Here's how the part is built. I have some questions about the finished solid (model axes, mm). A direction names the side the tool comes from. Round coordinates to 2 decimals unless told otherwise and drop trailing zeros. Order: outer loops, then holes, each group sorted by start corner. A loop starts at its lowest first (then second) coordinate and runs counter-clockwise, first axis right, second up. Notation, with made-up numbers: (31, 60) -> (75, 60) arc R26 cw to (75, 95) -> close; hole circle Ø4 at (24.25, 15.25). An arc over 180 degrees is marked (long way). Use a Markdown table: item, result. Add a question column.
from build123d import *

# Parameters (mm, degrees)
ESQUISSE11_R                 = 10
ENL_V_MAT_EXTRU_4_DEPTH      = 6.2
ESQUISSE12_R                 = 1.65
ENL_V_MAT_EXTRU_5_DEPTH      = 66.664775353
ESQUISSE14_R                 = 2.85
ENL_V_MAT_EXTRU_8_DEPTH      = 3.6
R_P_TITION_CIRCULAIRE7_COUNT = 3


with BuildPart() as part:
    # Esquisse1 → Révolution1 (revolve)
    with BuildSketch(Plane.XY, mode=Mode.PRIVATE) as r_volution1_sk:
        with BuildLine():
            Line((-45.5, 158.120727786), (-45.5, 145.030169275))
            ThreePointArc((-45.5, 145.030169275), (-23.015367368, 150.247438797), (0, 152))
            Line((0, 152), (0, 158.120727786))
            Line((0, 158.120727786), (-45.5, 158.120727786))
        make_face()
    revolve(r_volution1_sk.sketch.rotate(Axis((0, 0, 0), (0, 1, 0)), 270), axis=Axis((0, 0, 0), (0, 1, 0)))

    # Esquisse11 → Enlèv. mat.-Extru.4 (cut)
    with BuildSketch(Plane(origin=(0, 158.120727786, 0), x_dir=(1, 0, 0), z_dir=(0, 1, 0))):
        with Locations(Location((0, 35, 0), (0, 0, 270))):
            Circle(ESQUISSE11_R)
    enl_v_mat_extru_4 = extrude(amount=-ENL_V_MAT_EXTRU_4_DEPTH, mode=Mode.SUBTRACT)

    # Esquisse12 → Enlèv. mat.-Extru.5 (cut, through all)
    with BuildSketch(Plane(origin=(0, 158.120727786, 0), x_dir=(1, 0, 0), z_dir=(0, 1, 0))):
        with Locations(Location((-30.310889132, 17.5, 0), (0, 0, 270))):
            Circle(ESQUISSE12_R)
    enl_v_mat_extru_5 = extrude(amount=-ENL_V_MAT_EXTRU_5_DEPTH, mode=Mode.SUBTRACT)

    # Esquisse14 → Enlèv. mat.-Extru.8 (cut)
    with BuildSketch(Plane(origin=(0, 147.120727786, 0), x_dir=(1, 0, 0), z_dir=(0, 1, 0))):
        with Locations(Location((-30.310889132, 17.5, 0), (0, 0, 134.033255464))):
            Circle(ESQUISSE14_R)
    enl_v_mat_extru_8 = extrude(amount=ENL_V_MAT_EXTRU_8_DEPTH, mode=Mode.SUBTRACT)

    # Répétition circulaire7: Enlèv. mat.-Extru.4, Enlèv. mat.-Extru.5, Enlèv. mat.-Extru.8 ×3 about axis
    r_p_tition_circulaire7_axis = Axis((0, 0, 0), (0, 1, 0))
    add([enl_v_mat_extru_4.rotate(r_p_tition_circulaire7_axis, i * 360 / R_P_TITION_CIRCULAIRE7_COUNT) for i in range(1, R_P_TITION_CIRCULAIRE7_COUNT)], mode=Mode.SUBTRACT)
    add([enl_v_mat_extru_5.rotate(r_p_tition_circulaire7_axis, i * 360 / R_P_TITION_CIRCULAIRE7_COUNT) for i in range(1, R_P_TITION_CIRCULAIRE7_COUNT)], mode=Mode.SUBTRACT)
    add([enl_v_mat_extru_8.rotate(r_p_tition_circulaire7_axis, i * 360 / R_P_TITION_CIRCULAIRE7_COUNT) for i in range(1, R_P_TITION_CIRCULAIRE7_COUNT)], mode=Mode.SUBTRACT)


solid = part.part
(1) I'm going to push flat-ended pins straight in: P1, Ø1, axis at x = -18, y = 153, coming from the +Z side; P2, Ø1.5, axis at x = 6.5, y = 152.5, coming from the +Z side; P3, Ø6, axis at x = -31, z = 19, coming from the +Y side. Where does each tip first touch, or does it pass through?
(2) If we mould it in two halves opening along X, with no side actions, what happens to faces 4 (the cylindrical face through (0.08, 149.33, 37.85)), 5 (the flat face through (-1, 158.121, -1)), 6 (the cylindrical face through (27.686, 151.484, 36.107))? For each: pulls with the +X half, pulls with the -X half, needs draft (parallel to the pull), parting line crosses it, or undercut.
(3) I want a section at B-B on z = 17.5. List the corners of the cut face in (x, y) for me.
(4) I want a section at D-D on z = 0. List the corners of the cut face in (x, y) for me.
(5) Please list where these lines run through material, in increasing order: probe 1 along X at (y, z) = (152.75, -17.5); probe 2 along Z at (x, y) = (-8, 155.5); probe 3 along X at (y, z) = (154.5, 35). Write a range as from..to.
(6) I want a section at C-C on y = 156. List the corners of the cut face in (x, z) for me (3 decimals).
(7) I want a section at A-A on y = 148.5. List the corners of the cut face in (x, z) for me.
(8) On a 3-axis mill with a long thin cutter (end or side, diameter ignored), from which of +Z, -Z, +X, -X, +Y, -Y can I reach the whole of each face in a straight line? I mean faces 1 (the flat face through (-29, 150.721, -19)), 2 (the cylindrical face through (0, 155, -45)), 3 (the cylindrical face through (31, 154, -16)). Say none if no direction works.
Output:
| question | item | result |
|---|---|---|
| 1 | P1 | z = 42 |
| 1 | P2 | z = 45.14 |
| 1 | P3 | y = 151.92 |
| 2 | face 4 | undercut |
| 2 | face 5 | needs draft |
| 2 | face 6 | parting line crosses it |
| 3 | outline | (-42, 145.03) arc R150.99 cw to (42, 145.03) -> (42, 158.12) -> (40.31, 158.12) -> (40.31, 151.92) -> (20.31, 151.92) -> (20.31, 158.12) -> (-20.31, 158.12) -> (-20.31, 151.92) -> (-40.31, 151.92) -> (-40.31, 158.12) -> (-42, 158.12) -> close |
| 4 | outline | (-45.5, 145.03) arc R152 cw to (45.5, 145.03) -> (45.5, 158.12) -> (-45.5, 158.12) -> close |
| 5 | probe 1 | -42..-31.96, -28.66..28.66, 31.96..42 |
| 5 | probe 2 | -44.79..-41, -29..44.79 |
| 5 | probe 3 | -29.07..-1.65, 1.65..29.07 |
| 6 | outline | circle Ø91 at (0, 0); hole circle Ø20 at (-30.311, 17.5); hole circle Ø3.3 at (-30.311, -17.5); hole circle Ø20 at (0, -35); hole circle Ø3.3 at (0, 35); hole circle Ø20 at (30.311, 17.5); hole circle Ø3.3 at (30.311, -17.5) |
| 7 | outline | circle Ø91 at (0, 0); hole (-28.66, -15.18) arc R2.85 ccw (long way) to (-27.47, -17.23) arc R32.43 ccw to (27.47, -17.23) arc R2.85 ccw (long way) to (28.66, -15.18) arc R32.43 ccw to (1.19, 32.41) arc R2.85 ccw (long way) to (-1.19, 32.41) arc R32.43 ccw to start |
| 8 | face 1 | -Y |
| 8 | face 2 | +Y |
| 8 | face 3 | +Y, -Y |
